```python
from build123d import *

# Parameters (mm, degrees)
SKETCH1_R             = 45
SKETCH1_R_2           = 22.5
BOSS_EXTRUDE1_DEPTH   = 31.65
SKETCH1_R_3           = 56.25
SKETCH1_R_4           = 28.15
BOSS_EXTRUDE1_2_DEPTH = 31.65
BOSS_EXTRUDE2_DEPTH   = 12.5
CUT_EXTRUDE1_DEPTH    = 5
CUT_EXTRUDE2_DEPTH    = 64.3
FILLET1_R             = 10


with BuildPart() as part:
    # Sketch1 → Boss-Extrude1 (new body, symmetric)
    with BuildSketch(Plane(origin=(0, 0, 0), x_dir=(1, 0, 0), z_dir=(0, 1, 0))):
        Circle(SKETCH1_R)
        Circle(SKETCH1_R_2, mode=Mode.SUBTRACT)
    extrude(amount=BOSS_EXTRUDE1_DEPTH, both=True)



with BuildPart() as body_2:
    # Sketch1 → Boss-Extrude1 2 (new body, symmetric)
    with BuildSketch(Plane(origin=(0, 0, 0), x_dir=(1, 0, 0), z_dir=(0, 1, 0))):
        with Locations((0, 300)):
            Circle(SKETCH1_R_3)
        with Locations((0, 300)):
            Circle(SKETCH1_R_4, mode=Mode.SUBTRACT)
    extrude(amount=BOSS_EXTRUDE1_2_DEPTH, both=True)


with BuildPart() as part_1:
    add(part.part)

    add(body_2.part)  # Boss-Extrude2 merges body 2
    # Sketch2 → Boss-Extrude2 (add, symmetric)
    with BuildSketch(Plane(origin=(0, 0, 0), x_dir=(1, 0, 0), z_dir=(0, 1, 0))):
        with BuildLine():
            Line((56.210435304, 297.890625), (44.968348244, -1.6875))
            ThreePointArc((44.968348244, -1.6875), (0, 45), (-44.968348244, -1.6875))
            Line((-44.968348244, -1.6875), (-56.210435304, 297.890625))
            ThreePointArc((-56.210435304, 297.890625), (0, 243.75), (56.210435304, 297.890625))
        make_face()
    extrude(amount=BOSS_EXTRUDE2_DEPTH, both=True)

    # Sketch3 → Cut-Extrude1 (cut)
    with BuildSketch(Plane(origin=(0, 12.5, 0), x_dir=(1, 0, 0), z_dir=(0, 1, 0))):
        with BuildLine():
            Line((22.255863805, 59.73892388), (28.619814412, 229.324907336))
            ThreePointArc((28.619814412, 229.324907336), (0, 223.75), (-28.619814412, 229.324907336))
            Line((-28.619814412, 229.324907336), (-22.255863805, 59.73892388))
            ThreePointArc((-22.255863805, 59.73892388), (0, 63.75), (22.255863805, 59.73892388))
        make_face()
    cut_extrude1 = extrude(amount=-CUT_EXTRUDE1_DEPTH, mode=Mode.SUBTRACT)

    # Mirror1: Cut-Extrude1 across plane
    add(cut_extrude1.mirror(Plane.ZX), mode=Mode.SUBTRACT)

    # Sketch4 → Cut-Extrude2 (cut, through all)
    with BuildSketch(Plane(origin=(0, 31.65, 0), x_dir=(1, 0, 0), z_dir=(0, 1, 0))):
        with BuildLine():
            Line((-6.3, 272.564029086), (-6.3, 264.864029086))
            Line((-6.3, 264.864029086), (6.3, 264.864029086))
            Line((6.3, 264.864029086), (6.3, 272.564029086))
            ThreePointArc((6.3, 272.564029086), (0, 328.15), (-6.3, 272.564029086))
        make_face()
    extrude(amount=-CUT_EXTRUDE2_DEPTH, mode=Mode.SUBTRACT)

    # Fillet1
    fillet1_edges = [part_1.edges().sort_by_distance(p)[0] for p in [
        (-45, -31.65, 0),
        (-56.25, 31.65, -300),
        (-56.25, -31.65, -300),
        (-45, 31.65, 0),
    ]]
    fillet(fillet1_edges, radius=FILLET1_R)


solid = part_1.part
```
Design review of the part built by this model. Coordinates are the model's own, in mm. A direction names the side the tool comes from. Give positions to 0.01 mm unless a question says otherwise; leave off trailing zeros. Order: outer loops, then holes, each group sorted by start corner. A loop starts at its lowest first (then second) coordinate and runs counter-clockwise, first axis right, second up. Notation, with made-up numbers: (38, -28.75) -> (80, -28.75) arc R31 cw to (80, -2.75) -> close; hole circle Ø9 at (-1, -5.5). An arc over 180 degrees is marked (long way). Write item = value, one per line. Start each with the question number.
(1) We need section D-D on z = -217. Write out the cut boundary in (x, y).
(2) We need section A-A on y = 18. Write out the cut boundary in (x, z).
(3) For faces 1 (the face through (0, 0, -264.864)), 2 (the face through (-25.482, -10.035, -145.719)), 3 (the face through (0, 7.5, -146)), 4 (the face through (-7.32, 0.3, -355.77)), list the 3-axis set-ups (+Z, -Z, +X, -X, +Y, -Y) from which the entire face can be reached by the end or side of a thin tool; tool diameter is ignored.
(4) To check wall thickness, follow line 1 along Z through (x, y) = (0, 18.5); line 2 along Z through (x, y) = (-12.5, 18.5); line 3 along X through (y, z) = (18, 0). State the ranges of each line that lie inside material, in increasing order.
(5) Mouldability with a two-part tool opening along X and no side actions: class faces 5 (the face through (10.382, -0.443, 19.961)), 6 (the face through (-6.3, 0, -269)), 7 (the face through (0, 31.65, 23)), 8 (the face through (50.67, 0.18, -150.2)) as +X half, -X half, draft (parallel to the pull), parting line (faces both ways), or undercut.
(6) We need section B-B on y = -2.5. Write out the cut boundary in (x, z), plus the area to 3 significant figures.
(7) For pin 1 (10 mm diameter, centred on x = -2.5, y = -14, fed in from -Z); pin 2 (10 mm diameter, centred on y = -14, z = -103.5, fed in from -X); pin 3 (1 mm diameter, centred on x = -4, z = -157, fed in from +Y), all flat-tipped, find the tip position at first contact; note any pin that passes through.
(8) We need section C-C on x = 0. State how many separate pieces and enclosed holes the cut face has, plus the area to 3 significant figures.
Numbers:
q1.outline = (-53.17, -12.5) -> (-28.16, -12.5) -> (-28.16, -7.5) -> (28.16, -7.5) -> (28.16, -12.5) -> (53.17, -12.5) -> (53.17, 12.5) -> (28.16, 12.5) -> (28.16, 7.5) -> (-28.16, 7.5) -> (-28.16, 12.5) -> (-53.17, 12.5) -> close
q2.outline = circle Ø112.5 at (0, -300); circle Ø90 at (0, 0); hole circle Ø45 at (0, 0); hole (-6.3, -272.56) arc R28.15 ccw (long way) to (6.3, -272.56) -> (6.3, -264.86) -> (-6.3, -264.86) -> close
q3.face_1 = +Y, -Y
q3.face_2 = -Y
q3.face_3 = +Y
q3.face_4 = none
q4.line_1 = -356.25 to -328.15, -264.86 to -243.75, -45 to -22.5, 22.5 to 45
q4.line_2 = -354.84 to -325.22, -274.78 to -245.16, -43.23 to -18.71, 18.71 to 43.23
q4.line_3 = -45 to -22.5, 22.5 to 45
q5.face_5 = undercut
q5.face_6 = undercut
q5.face_7 = draft
q5.face_8 = +X half
q6.outline = (-56.21, -297.89) arc R56.25 ccw (long way) to (56.21, -297.89) -> (44.97, 1.69) arc R45 ccw to (-44.97, 1.69) -> close; hole circle Ø45 at (0, 0); hole (-6.3, -272.56) arc R28.15 ccw (long way) to (6.3, -272.56) -> (6.3, -264.86) -> (-6.3, -264.86) -> close
q6.area = 34,400 mm^2
q7.pin_1 = -356.25
q7.pin_2 = -49.09
q7.pin_3 = 7.5
q8.separate_pieces = 3
q8.enclosed_holes = 0
q8.area = 9,160 mm^2
